Design review of the part built by this model. Coordinates are the model's own, in mm. Coordinates: 2 decimals unless noted, no trailing zeros. Order: outer loops, then holes, each group sorted by start corner. A loop starts at its lowest first (then second) coordinate and runs counter-clockwise, first axis right, second up. Notation, with made-up numbers: M -3,3 L 16,3 A23 cw 16,36 Z; hole C -10,-33.75 d1. An arc over 180 degrees is marked long. Answer as a JSON object with one key per item and string values.
from build123d import *

# Parameters (mm, degrees)
SKETCH1_W           = 250
SKETCH1_H           = 100
SKETCH1_R           = 5
BOSS_EXTRUDE1_DEPTH = 10
FILLET1_R           = 0.2


with BuildPart() as part:
    # Sketch1 → Boss-Extrude1 (new body)
    with BuildSketch(Plane(origin=(0, 0, 0), x_dir=(1, 0, 0), z_dir=(0, 1, 0))):
        Rectangle(SKETCH1_W, SKETCH1_H)
        with Locations(Location((100, 25, 0), (0, 0, 270))):
            Circle(SKETCH1_R, mode=Mode.SUBTRACT)
        with Locations(Location((100, -25, 0), (0, 0, 90))):
            Circle(SKETCH1_R, mode=Mode.SUBTRACT)
        with Locations(Location((-100, -25, 0), (0, 0, 270))):
            Circle(SKETCH1_R, mode=Mode.SUBTRACT)
        with Locations(Location((-100, 25, 0), (0, 0, 90))):
            Circle(SKETCH1_R, mode=Mode.SUBTRACT)
    extrude(amount=BOSS_EXTRUDE1_DEPTH)

    # Fillet1
    fillet1_edges = [part.edges().sort_by_distance(p)[0] for p in [
        (-125, 10, 0),
        (0, 10, 50),
        (125, 10, 0),
        (0, 0, 50),
        (-125, 0, 0),
        (0, 0, -50),
        (125, 0, 0),
        (0, 10, -50),
        (125, 5, 50),
        (-125, 5, 50),
        (-125, 5, -50),
        (125, 5, -50),
    ]]
    fillet(fillet1_edges, radius=FILLET1_R)


solid = part.part
1) Add section A-A (x = 100). State the section outline as (y, z) points.
Taken from the geometry:
{"outline": "M 0,-49.8 A0.2 ccw 0.2,-50 L 9.8,-50 A0.2 ccw 10,-49.8 L 10,-30 L 0,-30 Z; M 0,-20 L 10,-20 L 10,20 L 0,20 Z; M 0,30 L 10,30 L 10,49.8 A0.2 ccw 9.8,50 L 0.2,50 A0.2 ccw 0,49.8 Z"}
2) To check wall thickness, follow L1, parallel to X at y = 7.75, z = 25; L2, parallel to X at y = 1, z = -26.5; L3, parallel to Z at x = 104.5, y = 4.25. State the ranges of each line that lie inside material, in increasing order.
Taken from the geometry:
{"L1": "x = -125 to -105, -95 to 95, 105 to 125", "L2": "x = -125 to -104.77, -95.23 to 95.23, 104.77 to 125", "L3": "z = -50 to -27.18, -22.82 to 22.82, 27.18 to 50"}
3) Add section B-B (z = -25). State the section outline as (x, y) points, and give its area (3 significant figures).
Taken from the geometry:
{"outline": "M -125,0.2 A0.2 ccw -124.8,0 L -105,0 L -105,10 L -124.8,10 A0.2 ccw -125,9.8 Z; M -95,0 L 95,0 L 95,10 L -95,10 Z; M 105,0 L 124.8,0 A0.2 ccw 125,0.2 L 125,9.8 A0.2 ccw 124.8,10 L 105,10 Z", "area": "2,300 mm2"}
4) Mouldability with a two-part tool opening along X and no side actions: class faces 1 (the flat face through (-125, 5, 1)), 2 (the flat face through (-2, 10, -1)), 3 (the cylindrical face through (100, 5, -30)), 4 (the flat face through (125, 5, 1)) as released by +X, released by -X, zero draft, split by the parting line, or undercut.
Taken from the geometry:
{"face 1": "released by -X", "face 2": "zero draft", "face 3": "undercut", "face 4": "released by +X"}
5) Insertion check: pin 1 Ø6 at (x, z) = (100, -25) entering from +Y. The pin has a flat end and moves straight along its axis. Give the tip position at first contact, or say it passes through.
Taken from the geometry:
{"pin 1": "passes through"}
